Geometry check sheet. Reference: the model listing, model coordinates, mm. A direction names the side the tool comes from. Round coordinates to 2 decimals unless told otherwise and drop trailing zeros. Order: outer loops, then holes, each group sorted by start corner. A loop starts at its lowest first (then second) coordinate and runs counter-clockwise, first axis right, second up. Notation, with made-up numbers: (19, 34) - (53, 34) arc R30 cw to (53, 64) - close; hole circle Ø1 at (47.5, 75.5). An arc over 180 degrees is marked (long way). Use a Markdown table: item, result. Add a question column.
(1) Section check C-C on y = 3.5. Record the boundary of the cut face in (x, z), then the cut area to 3 significant figures.
(2) Mould release check, pull along X, two halves, no side actions. Record for faces 1 (the face through (0.404, 3.62, 14.465)), 2 (the face through (0.2, 3, 4.5)), 3 (the face through (12, 1, 13)), 4 (the face through (-12, 1, 13)): released by +X, released by -X, zero draft, split by the parting line, or undercut.
(3) Section check A-A on x = 0. Record the boundary of the cut face in (y, z), then the cut area to 3 significant figures.
(4) Section check D-D on z = 18.25. Record the boundary of the cut face in (x, y).
(5) Section check B-B on z = 9.75. Record the boundary of the cut face in (x, y).
(6) Gauge pin test, flat ends, axial feed: P1, Ø4, axis at y = 3, z = 12.5, coming from the -X side; P2, Ø1.5, axis at y = 5, z = 18.5, coming from the +X side; P3, Ø4, axis at x = -3, y = 5.5, coming from the -Z side. Record the tip position at first contact, or that the pin passes through.
(7) Access from +Z, -Z, +X, -X, +Y, -Y to the whole of each face (thin tool, end or side, straight path). Record for faces 5 (the face through (0, 3, 22)), 6 (the face through (2, 6, 17)).
(8) Thickness scan on line 1 along X through (y, z) = (6.25, 11.25); line 2 along Z through (x, y) = (0, 2.25); line 3 along Y through (x, z) = (-2.5, 18.25). Record the ranges inside material, lowest first. Write a range as [from, to].
```python
from build123d import *

# Parameters (mm, degrees)
BOSS_EXTRUDE1_DEPTH = 22
SKETCH2_R           = 5.625
BOSS_EXTRUDE2_DEPTH = 1.14
SKETCH3_R           = 3.1
CUT_EXTRUDE3_DEPTH  = 27.057236999
CUT_EXTRUDE4_DEPTH  = 26.768197453


with BuildPart() as part:
    # Sketch1 → Boss-Extrude1 (new body)
    with BuildSketch(Plane.XY):
        Polygon((-12, 0), (12, 0), (12, 1.6), (7.6, 6), (-7.6, 6), (-12, 1.6), align=None)
    extrude(amount=BOSS_EXTRUDE1_DEPTH)

    # Sketch2 → Boss-Extrude2 (add)
    with BuildSketch(Plane(origin=(0, 6, 0), x_dir=(1, 0, 0), z_dir=(0, 1, 0))):
        with Locations(Location((0, -11.391064781, 0), (0, 0, 180))):
            Circle(SKETCH2_R)
    extrude(amount=BOSS_EXTRUDE2_DEPTH)

    # Sketch3 → Cut-Extrude3 (cut, through all)
    with BuildSketch(Plane(origin=(0, 7.14, 0), x_dir=(1, 0, 0), z_dir=(0, 1, 0))):
        with Locations(Location((0, -11.391064781, 0), (0, 0, 180))):
            Circle(SKETCH3_R)
    extrude(amount=-CUT_EXTRUDE3_DEPTH, mode=Mode.SUBTRACT)

    # Sketch4 → Cut-Extrude4 (cut, through all)
    with BuildSketch(Plane(origin=(0, 6, 0), x_dir=(1, 0, 0), z_dir=(0, 1, 0))):
        with BuildLine():
            Line((-12, -3.648677946), (-12, 0))
            Line((-12, 0), (12, 0))
            Line((12, 0), (12, -3.648677946))
            ThreePointArc((12, -3.648677946), (0, -4.5), (-12, -3.648677946))
        make_face()
    extrude(amount=-CUT_EXTRUDE4_DEPTH, mode=Mode.SUBTRACT)


solid = part.part
```
Check sheet entries:
| question | item | result |
|---|---|---|
| 1 | outline | (-10.1, 3.9) arc R85 cw to (10.1, 3.9) - (10.1, 22) - (-10.1, 22) - close; hole circle Ø6.2 at (0, 11.39) |
| 1 | area | 327 mm2 |
| 2 | face 1 | undercut |
| 2 | face 2 | undercut |
| 2 | face 3 | released by +X |
| 2 | face 4 | released by -X |
| 3 | outline | (0, 4.5) - (6, 4.5) - (6, 5.77) - (7.14, 5.77) - (7.14, 8.29) - (0, 8.29) - close; (0, 14.49) - (7.14, 14.49) - (7.14, 17.02) - (6, 17.02) - (6, 22) - (0, 22) - close |
| 3 | area | 73.6 mm2 |
| 4 | outline | (-12, 0) - (12, 0) - (12, 1.6) - (7.6, 6) - (-7.6, 6) - (-12, 1.6) - close |
| 5 | outline | (-12, 0) - (-2.63, 0) - (-2.63, 7.14) - (-5.38, 7.14) - (-5.38, 6) - (-7.6, 6) - (-12, 1.6) - close; (2.63, 0) - (12, 0) - (12, 1.6) - (7.6, 6) - (5.38, 6) - (5.38, 7.14) - (2.63, 7.14) - close |
| 6 | P1 | stops at x = -12 |
| 6 | P2 | stops at x = 9.35 |
| 6 | P3 | stops at z = 4.35 |
| 7 | face 5 | +Z, +X, -X, +Y, -Y |
| 7 | face 6 | +Y |
| 8 | line 1 | x = [-5.62, -3.1], [3.1, 5.62] |
| 8 | line 2 | z = [4.5, 8.29], [14.49, 22] |
| 8 | line 3 | y = [0, 6] |
